Build history of the part. All positions in model axes, mm. A direction names the side the tool comes from. Give positions to 0.01 mm unless a question says otherwise; leave off trailing zeros. Order: outer loops, then holes, each group sorted by start corner. A loop starts at its lowest first (then second) coordinate and runs counter-clockwise, first axis right, second up. Notation, with made-up numbers: M 26,8 L 66,8 A26 cw 66,37 Z; hole C -0.5,-31 d6. An arc over 180 degrees is marked long. Use CSV: the item, a comma, the result in double quotes. Start each with the question number.
Item 1: Pin check, flat tips, straight feed: P1, Ø2, axis at x = 1.5, z = 13.5, coming from the +Y side; P2, Ø1, axis at x = 1, z = 14.5, coming from the -Y side; P3, Ø1.6, axis at x = -31, y = -1, coming from the +Z side. Stop position of each tip, or through.
Item 2: Band-saw the part on D-D on y = 8. Write the cut outline in (x, z).
Item 3: Band-saw the part on A-A on y = 17. Write the cut outline in (x, z), plus the area to 3 significant figures.
Item 4: Band-saw the part on B-B on x = -17.5. Write the cut outline in (y, z).
Item 5: Wall check: line 1 along Z through (x, y) = (-5, 33.5); line 2 along X through (y, z) = (14.5, 4.25); line 3 along Y through (x, z) = (-5, 25.5). Give the ranges that are in metal, low to high.
Item 6: Two-plate mould, pull along X, no slides. Class faces 1 (the flat face through (2, 4, 15)), 2 (the flat face through (-4.8, -1, 14)), 3 (the flat face through (-32, 6.8, 2)): pulls with the +X half, pulls with the -X half, needs draft (parallel to the pull), parting line crosses it, or undercut.
Item 7: Band-saw the part on C-C on z = 14.5. Give the number of separate pieces and of enclosed holes in the cut face, plus the area to 3 significant figures.
Item 8: Which spindle directions (+Z, -Z, +X, -X, +Y, -Y) get a long thin tool onto all of the face, cutting with end or side? Do faces 4 (the flat face through (-32, -1, 14)), 5 (the flat face through (-2.6, -1, 15)), 6 (the flat face through (-20, 4, 10)), 7 (the flat face through (-2, 18, 10.9)). Say none if no direction does.
Autodesk Inventor part; units mm, degrees
ref_plane "YZ Plane" through (0, 0, 0) normal (1, 0, 0) x (0, 1, 0)
ref_plane "XZ Plane" through (0, 0, 0) normal (0, 1, 0) x (-1, 0, 0)
ref_plane "XY Plane" through (0, 0, 0) normal (0, 0, 1) x (1, 0, 0)
sketch "Sketch1" plane through (0, 0, 0) normal (0, 0, 1) x (1, 0, 0)
  line L0 (0, 0) -> (0, 35)
  line L1 (0, 35) -> (-5.8, 35)
  line L2 (-6.8, 34) -> (-6.8, 29.4142)
  line L3 (0, 0) -> (-35, 0)
  line L4 (0, 0) -> (35, 0) construction
  line L5 (-35, 0) -> (-35, 5.8)
  line L6 (-34, 6.8) -> (-29.4142, 6.8)
  line L7 (-28.7071, 7.0929) -> (-7.0929, 28.7071)
  arc A0 (-5.8, 35) -> (-6.8, 34) centre (-5.8, 34) ccw
  arc A1 (-7.0929, 28.7071) -> (-6.8, 29.4142) centre (-7.8, 29.4142) ccw
  arc A2 (-29.4142, 6.8) -> (-28.7071, 7.0929) centre (-29.4142, 7.8) ccw
  arc A3 (-34, 6.8) -> (-35, 5.8) centre (-34, 5.8) ccw
  point P0 (-6.8, 35)
  point P1 (-6.8, 29)
  point P2 (-35, 6.8)
  point P3 (-29, 6.8)
  dimension "d0" = 35
  dimension "d1" = 6.8
  dimension "d2" = 90
  dimension "d3" = 6
  dimension "d4" = 35
  dimension "d5" = 180
  dimension "d6" = 6.8
  dimension "d7" = 6
  dimension "d8" = 90
  dimension "d9" = 1
extrude "Extrusion1" add sketch "Sketch1" along normal blind 29
ref_plane "Work Plane1" through (0, 0, 25.6) normal (0, 0, 1) x (1, 0, 0)
sketch "Sketch2" plane through (0, 0, 25.6) normal (0, 0, 1) x (1, 0, 0)
  line L0 (0, 0) -> (0, 35)
  line L1 (0, 35) -> (-5.8, 35)
  arc A0 (-5.8, 35) -> (-6.8, 34) centre (-5.8, 34) ccw
  line L2 (-6.8, 34) -> (-6.8, 29.4142)
  arc A1 (-7.0929, 28.7071) -> (-6.8, 29.4142) centre (-7.8, 29.4142) ccw
  line L3 (-7.0929, 28.7071) -> (-28.7071, 7.0929)
  arc A2 (-29.4142, 6.8) -> (-28.7071, 7.0929) centre (-29.4142, 7.8) ccw
  line L4 (-29.4142, 6.8) -> (-34, 6.8)
  arc A3 (-34, 6.8) -> (-35, 5.8) centre (-34, 5.8) ccw
  line L5 (-35, 5.8) -> (-35, 0)
  line L6 (-35, 0) -> (0, 0)
  line L7 (0, 0) -> (-4, 0)
  line L8 (-35, 0) -> (0, 0)
  line L9 (-4, 0) -> (-4, 35)
  line L10 (-4, 0) -> (-4, 4)
  line L11 (-4, 4) -> (-35, 4)
  line L12 (-35, 5.8) -> (-35, 0)
  line L13 (-4, 4) -> (-36.3789, 4)
  line L14 (-36.3789, 4) -> (-36.3789, 37.1754)
  line L15 (-36.3789, 37.1754) -> (-4, 37.1754)
  line L16 (-4, 37.1754) -> (-4, 4)
  dimension "d13" = 4
extrude "Extrusion2" cut sketch "Sketch2" against normal blind 22.2 contours L9 L11 L5 A3 L4 A2 L3 A1 L2 A0 L1
sketch "Sketch3" plane through (-35, 4, 25.6) normal (0, 1, 0) x (1, 0, 0)
  line L0 (0, 0) -> (0, 22.2)
  line L1 (0, 11.1) -> (9, 11.1)
  line L2 (9, 11.1) -> (12.6, 11.1)
  arc A0 (12.6, 14.7) -> (12.6, 7.5) centre (12.6, 11.1) ccw
  line L3 (17.8, 11.1) -> (25, 11.1)
  line L4 (25, 11.1) -> (21.4, 11.1)
  arc A1 (21.4, 7.5) -> (21.4, 14.7) centre (21.4, 11.1) ccw
  line L5 (12.6, 14.7) -> (21.4, 14.7)
  line L6 (12.6, 7.5) -> (21.4, 7.5)
  point P0 (35, 25.6)
  dimension "d16" = 9
  dimension "d17" = 3.6
  dimension "d18" = 16
  dimension "d19" = 3.6
extrude "Extrusion3" cut sketch "Sketch3" against normal blind 22.2
fillet "Fillet1" radius 1 1 edges at (-4, 4, 14.5)
sketch "Sketch4" plane through (0, 0, 0) normal (0, 0, -1) x (-1, 0, 0)
  line L0 (5, 4) -> (35, 4)
  line L1 (4, 35) -> (4, 5)
  line L2 (0, 0) -> (0, 2)
  line L3 (0, 0) -> (0, 35)
  line L4 (0, 2) -> (0, 0)
  line L5 (0, 2) -> (2, 2)
  dimension "d23" = 2
  dimension "d24" = 2
  dimension "d25" = 2
pattern_circular "Circular Pattern1" count 2 over 270 about axis through (-2, 2, 0) along (0, 0, 1) of "Extrusion3"
sketch "Sketch5" plane through (-35, 0, 0) normal (0, -1, 0) x (1, 0, 0)
  line L0 (0, 25.6) -> (0, 3.4)
  line L1 (0, 14.5) -> (3, 14.5)
  line L2 (0, 14.5) -> (3, 14.5) construction
  line L3 (3, 14.5) -> (3, 11.75)
  line L4 (3, 11.75) -> (3, 17.25)
  line L5 (3, 17.25) -> (5.2, 17.25)
  line L6 (5.2, 17.25) -> (5.2, 11.75)
  line L7 (5.2, 11.75) -> (3, 11.75)
  line L8 (35, 0) -> (35, 29)
  line L9 (35, 14.5) -> (32.4, 14.5)
  line L10 (32.4, 14.5) -> (32.4, 11.75)
  line L11 (32.4, 11.75) -> (30.2, 11.75)
  line L12 (30.2, 11.75) -> (30.2, 17.25)
  line L13 (30.2, 17.25) -> (32.4, 17.25)
  line L14 (32.4, 17.25) -> (32.4, 11.75)
  dimension "d29" = 3
  dimension "d30" = 0
  dimension "d31" = 2.75
  dimension "d32" = 5.5
  dimension "d33" = 2.2
  dimension "d34" = 2.6
  dimension "d35" = 2.75
  dimension "d36" = 2.2
  dimension "d37" = 5.5
extrude "Extrusion4" add sketch "Sketch5" along normal blind 2
sketch "Sketch7" plane through (-35, -2, 0) normal (0, -1, 0) x (1, 0, 0)
  point P0 (35, 0)
sketch "Sketch9" plane through (0, 0, 0) normal (1, 0, 0) x (0, 0, -1)
  line L0 (-10.9, 22.4) -> (-10.9, 13.6)
  arc A0 (-18.1, 13.6) -> (-10.9, 13.6) centre (-14.5, 13.6) ccw
  line L1 (-18.1, 13.6) -> (-18.1, 22.4)
  arc A1 (-10.9, 22.4) -> (-18.1, 22.4) centre (-14.5, 22.4) ccw
  line L2 (0, 0) -> (0, 35)
  line L3 (0, 35) -> (-29, 35)
  line L4 (-29, 0) -> (-29, 35)
  line L5 (0, 0) -> (-29, 0)
  line L6 (-11.75, 32) -> (-11.75, 29.8)
  line L7 (-11.75, 32) -> (-17.25, 32)
  line L8 (-17.25, 32) -> (-17.25, 29.8)
  line L9 (-17.25, 29.8) -> (-11.75, 29.8)
  line L10 (-11.75, 29.8) -> (-11.75, 32)
  line L11 (-11.75, 2.6) -> (-17.25, 2.6)
  line L12 (-11.75, 4.8) -> (-17.25, 4.8)
  line L13 (-17.25, 4.8) -> (-17.25, 2.6)
  line L14 (-17.25, 2.6) -> (-11.75, 2.6)
  line L15 (-11.75, 2.6) -> (-11.75, 4.8)
extrude "Extrusion5" add sketch "Sketch9" along normal blind 2 contours L6 L9 L8 L7 | L11 L13 L12 L15
properties part number "30mm Bracket"
Model answer:
1,P1,"stops at y = 32"
1,P2,"stops at y = 2.6"
1,P3,"stops at z = 17.25"
2,outline,"M -27.8,0 L 0,0 L 0,29 L -27.8,29 L -27.8,25.6 L -4,25.6 L -4,3.4 L -27.8,3.4 Z"
3,outline,"M -18.8,0 L 0,0 L 0,10.9 L -4,10.9 L -4,3.4 L -18.8,3.4 Z; M -18.8,25.6 L -4,25.6 L -4,18.1 L 0,18.1 L 0,29 L -18.8,29 Z"
3,area,"188 mm^2"
4,outline,"M 0,0 L 18.3,0 L 18.3,3.4 L 4,3.4 L 4,10.9 L 0,10.9 Z; M 0,18.1 L 4,18.1 L 4,25.6 L 18.3,25.6 L 18.3,29 L 0,29 Z"
5,line 1,"z = 0 to 3.4, 25.6 to 29"
5,line 2,"x = -4 to 0"
5,line 3,"y = 0 to 4"
6,face 1,"pulls with the +X half"
6,face 2,"undercut"
6,face 3,"needs draft"
7,separate pieces,"3"
7,enclosed holes,"0"
7,area,"154 mm^2"
8,face 4,"+Z, -Z, -X, -Y"
8,face 5,"+Z, -Z, +X, -Y"
8,face 6,"-X, +Y"
8,face 7,"+X, -X"
